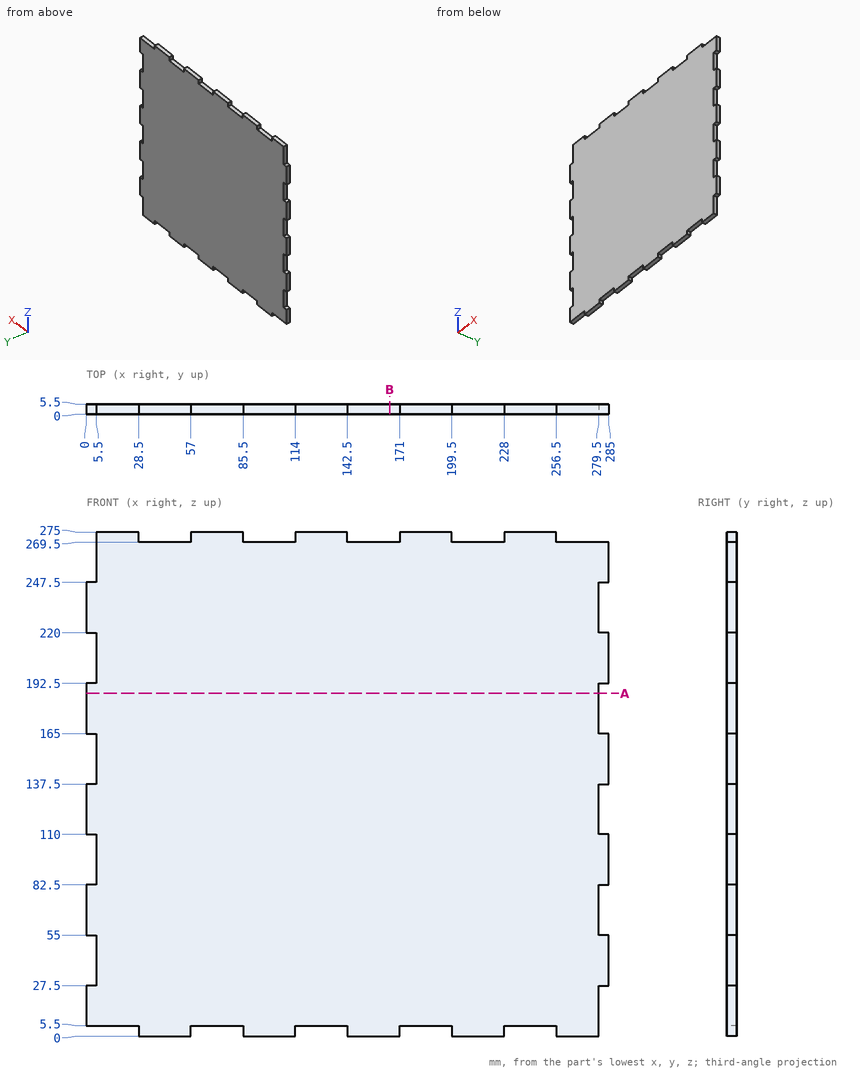
Could you check a few things on this drawing? It's one solid part, dimensions in mm from its lowest x, y, z. Give positions to 0.01 mm unless a question says otherwise; leave off trailing zeros. Order: outer loops, then holes, each group sorted by start corner. A loop starts at its lowest first (then second) coordinate and runs counter-clockwise, first axis right, second up. Notation, with made-up numbers: M 1,42.25 L 53,42.25 A27 cw 53,59.25 Z; hole C 42,25 d10. An arc over 180 degrees is marked long. Use one line per item in the form item = value.
Item 1: If we section it at A-A, the plane z = 187: Write out the boundary of the cut face in (x, y), and give its area (3 significant figures).
Values follow:
outline = M 0,0 L 279.5,0 L 279.5,5.5 L 0,5.5 Z
area = 1,540 mm^2
Item 2: Will these pins go through, and if not, where does the flat tip stop? pin 1 Ø1.6 at (x, y) = (282.5, 1.5) entering from +Z; pin 2 Ø2 at (x, y) = (245.5, 5) entering from -Z; pin 3 Ø3 at (y, z) = (1.5, 146) entering from -X.
Values follow:
pin_1 = 269.5
pin_2 = 5.5
pin_3 = 5.5
Item 3: If we section it at B-B, the plane x = 165.5: Write out the boundary of the cut face in (y, z), and give its area (3 significant figures).
Values follow:
outline = M 0,0 L 5.5,0 L 5.5,269.5 L 0,269.5 Z
area = 1,480 mm^2
Item 4: If I drill on line 1 along X through (y, z) = (3, 97.5); line 2 along X through (y, z) = (1.1, 167); line 3 along Z through (x, y) = (223, 2.05), over which ranges is the centre line in solid material (lowest first)? Write a range as [from, to].
Values follow:
line_1 = [5.5, 285]
line_2 = [0, 279.5]
line_3 = [0, 269.5]
